```python
from build123d import *

# Parameters (mm, degrees)
BOSS_EXTRUDE1_DEPTH = 5
CUT_EXTRUDE1_DEPTH  = 2


with BuildPart() as part:
    # Sketch1 → Boss-Extrude1 (new body)
    with BuildSketch(Plane.XY):
        Polygon((-73.645107518, -74.864510752), (-51.383851785, -74.864510752), (-51.383851785, -79.864510752), (-31.383851785, -79.864510752), (-31.383851785, -74.864510752), (22.715789763, -74.864510752), (22.715789763, -79.864510752), (42.715789763, -79.864510752), (42.715789763, -74.864510752), (76.354892482, -74.864510752), (76.354892482, -60.328664174), (71.354892482, -60.328664174), (71.354892482, -40.328664174), (76.354892482, -40.328664174), (76.354892482, -12.973595237), (71.354892482, -12.973595237), (71.354892482, 7.026404763), (76.354892482, 7.026404763), (76.354892482, 37.571193369), (71.355899646, 37.470840861), (71.355899646, 57.470840861), (76.354892482, 57.571193369), (76.354892482, 75.135489248), (42.715789763, 75.135489248), (42.715789763, 80.135489248), (22.715789763, 80.135489248), (22.715789763, 75.135489248), (-31.383851785, 75.135489248), (-31.383851785, 80.135489248), (-51.383851785, 80.135489248), (-51.383851785, 75.135489248), (-73.645107518, 75.135489248), (-73.645107518, 57.571193369), (-68.646114682, 57.470840861), (-68.646114682, 37.470840861), (-73.645107518, 37.571193369), (-73.645107518, 7.026404763), (-68.645107518, 7.026404763), (-68.645107518, -12.973595237), (-73.645107518, -12.973595237), (-73.645107518, -40.328664174), (-68.645107518, -40.328664174), (-68.645107518, -60.328664174), (-73.645107518, -60.328664174), align=None)
    extrude(amount=BOSS_EXTRUDE1_DEPTH)

    # Sketch2 → Cut-Extrude1 (cut)
    with BuildSketch(Plane.XY.offset(5)):
        with BuildLine():
            Line((-24.19666878, 43.178385546), (-25.33641237, 43.178385546))
            add(Edge.make_bspline(
                [(-25.33641237, 43.178385546), (-25.328984129, 43.329591339), (-25.314395262, 43.626555492), (-25.246075469, 44.059530809), (-25.148318572, 44.473386793), (-25.01010101, 44.864800481), (-24.838446802, 45.237232725), (-24.632597846, 45.58920421), (-24.38878016, 45.919372238), (-24.112258582, 46.22467604), (-23.811926663, 46.504756655), (-23.487873683, 46.746619964), (-23.147350298, 46.950972657), (-22.791389622, 47.121810306), (-22.415975577, 47.250043461), (-22.024514921, 47.345190554), (-21.615287769, 47.402436151), (-21.33646826, 47.40858943), (-21.194665575, 47.41171888)],
                knots=[0, 0, 0, 0, 0.000453872, 0.000891393, 0.001312835, 0.001728009, 0.002134376, 0.002541468, 0.002949043, 0.00336336, 0.003775633, 0.004179123, 0.004573978, 0.004965443, 0.005361289, 0.005761752, 0.006172633, 0.006597866, 0.006597866, 0.006597866, 0.006597866], degree=3))
            add(Edge.make_bspline(
                [(-21.194665575, 47.41171888), (-21.055407992, 47.408458766), (-20.781771816, 47.40205276), (-20.382403935, 47.347039882), (-20.002212038, 47.260877307), (-19.641939285, 47.139989939), (-19.304460136, 46.977486445), (-18.987239375, 46.782278234), (-18.686500433, 46.556509131), (-18.415784389, 46.290702437), (-18.16719793, 46.006939499), (-17.952741176, 45.703997677), (-17.769087697, 45.391108555), (-17.616006687, 45.065886223), (-17.503317269, 44.725268492), (-17.417762057, 44.374214356), (-17.369402584, 44.009090042), (-17.361980619, 43.76196054), (-17.358207242, 43.636318239)],
                knots=[0, 0, 0, 0, 0.000417607, 0.000820584, 0.001206914, 0.001585844, 0.001957948, 0.002327951, 0.002701938, 0.003083379, 0.003463911, 0.003832406, 0.004194997, 0.004551257, 0.004908462, 0.005269442, 0.005633919, 0.006010863, 0.006010863, 0.006010863, 0.006010863], degree=3))
            add(Edge.make_bspline(
                [(-17.358207242, 43.636318239), (-17.364327354, 43.459426074), (-17.376460178, 43.108745951), (-17.481165156, 42.592747282), (-17.642934479, 42.092348925), (-17.839142328, 41.689653506), (-18.037336959, 41.366794494), (-18.212160789, 41.09858631), (-18.421356469, 40.812559028), (-18.66300994, 40.505831861), (-18.933475694, 40.177466576), (-19.234700346, 39.827328424), (-19.568984994, 39.459136174), (-19.803601825, 39.207655081), (-19.925174389, 39.07734388)],
                knots=[0, 0, 0, 0, 0.000530199, 0.001051094, 0.001573224, 0.002104594, 0.002389938, 0.002709581, 0.003064778, 0.003452579, 0.003880929, 0.004340927, 0.00483807, 0.005372718, 0.005372718, 0.005372718, 0.005372718], degree=3))
            Line((-19.925174389, 39.07734388), (-23.10271846, 35.688641956))
            Line((-23.10271846, 35.688641956), (-17.195386729, 35.688641956))
            Line((-17.195386729, 35.688641956), (-17.195386729, 34.386077854))
            Line((-17.195386729, 34.386077854), (-25.824873909, 34.386077854))
            Line((-25.824873909, 34.386077854), (-20.899553396, 39.642127533))
            add(Edge.make_bspline(
                [(-20.899553396, 39.642127533), (-20.779636778, 39.767307103), (-20.549301497, 40.007751437), (-20.223519004, 40.358790178), (-19.930914675, 40.684452798), (-19.669594421, 40.984123988), (-19.44522713, 41.262187105), (-19.246119317, 41.509636458), (-19.08658703, 41.737345463), (-18.913448308, 42.001289977), (-18.745757576, 42.323551813), (-18.601658455, 42.717374057), (-18.513793148, 43.122784374), (-18.503252745, 43.396748909), (-18.497950832, 43.534555418)],
                knots=[0, 0, 0, 0, 0.000520043, 0.000998896, 0.001436661, 0.001833471, 0.002191472, 0.002508543, 0.002785952, 0.003025175, 0.003455296, 0.003872183, 0.004280329, 0.004693418, 0.004693418, 0.004693418, 0.004693418], degree=3))
            add(Edge.make_bspline(
                [(-18.497950832, 43.534555418), (-18.500257668, 43.621210778), (-18.504803999, 43.791991852), (-18.544927645, 44.042384178), (-18.60556291, 44.283919359), (-18.692449989, 44.517340349), (-18.807137303, 44.740300286), (-18.94674071, 44.953070571), (-19.107813226, 45.158770531), (-19.294144974, 45.35164107), (-19.498838203, 45.528284301), (-19.715080195, 45.684763125), (-19.943862002, 45.815533613), (-20.184219016, 45.922734303), (-20.435481148, 46.006827829), (-20.698134366, 46.065097531), (-20.97145294, 46.101682544), (-21.158083053, 46.10663254), (-21.253179197, 46.109154777)],
                knots=[0, 0, 0, 0, 0.000259807, 0.000512029, 0.000758843, 0.001005985, 0.001257437, 0.001509351, 0.001768409, 0.002040101, 0.00231246, 0.002578628, 0.002839591, 0.003101519, 0.003367006, 0.003633016, 0.003907552, 0.004192772, 0.004192772, 0.004192772, 0.004192772], degree=3))
            add(Edge.make_bspline(
                [(-21.253179197, 46.109154777), (-21.352496219, 46.106560231), (-21.547538451, 46.101464972), (-21.833901799, 46.065822734), (-22.10708162, 46.004333542), (-22.367765097, 45.920235323), (-22.616393308, 45.813342875), (-22.851757125, 45.680204258), (-23.07332818, 45.521332726), (-23.281522993, 45.341208422), (-23.473343717, 45.140665983), (-23.641879524, 44.917109831), (-23.789141518, 44.674621781), (-23.917626451, 44.413856126), (-24.021968527, 44.132446696), (-24.101699673, 43.831392453), (-24.164789088, 43.512000583), (-24.18586572, 43.291437561), (-24.19666878, 43.178385546)],
                knots=[0, 0, 0, 0, 0.000297928, 0.000585081, 0.00086406, 0.001136798, 0.001405713, 0.001674567, 0.001946354, 0.002222301, 0.00249943, 0.002777246, 0.003060416, 0.003349412, 0.003648067, 0.00395911, 0.004282927, 0.004623434, 0.004623434, 0.004623434, 0.004623434], degree=3))
        make_face()
    extrude(amount=-CUT_EXTRUDE1_DEPTH, mode=Mode.SUBTRACT)


solid = part.part
```
Check sheet for the modelled part. Datum: model origin and axes. Units: mm. A direction names the side the tool comes from. Round coordinates to 2 decimals unless told otherwise and drop trailing zeros. Write each loop counter-clockwise with the first axis right and the second up, starting at its lowest first coordinate (ties: lowest second). Pieces come first, ordered by that corner, then holes. Notation, with made-up numbers: (75, -0.5) -> (116, -0.5) arc R28 ccw to (116, 25.5) -> close; hole circle Ø9 at (71, 33.5). An arc over 180 degrees is marked (long way). One line per question, with ' | ' between items. Start each with the question number.
1. Release check for a two-part mould opening along Y. For faces 1 (the face through (-73.645, -67, 2)), 2 (the face through (74, 7.026, 2)), 3 (the face through (-42, -79.865, 2)) record: +Y half, -Y half, draft (parallel to the pull), parting line (faces both ways), or undercut.
2. Sectioned sample at A-A, the plane x = 6. Record the cut outline in (y, z), then the cut area to 3 significant figures.
3. Set-up check for faces 4 (the face through (59, -74.865, 2)), 5 (the face through (71.355, -50, 2)), 6 (the face through (-31.384, 78, 2)): record each of +Z, -Z, +X, -X, +Y, -Y from which the full face is reachable in a straight line by a thin tool's end or side.
4. Sectioned sample at B-B, the plane y = 53. Record the cut outline in (x, z).
5. Depth check by flat-ended pin: pin 1 (2 mm diameter, centred on x = -20, z = 3.5, fed in from -Y); pin 2 (2.5 mm diameter, centred on y = 76.5, z = 2, fed in from -X); pin 3 (1.5 mm diameter, centred on x = 67.5, z = 1.5, fed in from +Y). Enter the tip coordinate at first touch or a pass-through.
6. Scan lines: line 1 along Y through (x, z) = (-16.5, 0.3); line 2 along X through (y, z) = (-5.5, 2.45). Record each from-to range of solid material in increasing order. Write a range as from..to.
Taken from the geometry:
1) face 1: draft | face 2: undercut | face 3: -Y half
2) outline: (-74.86, 0) -> (75.14, 0) -> (75.14, 5) -> (-74.86, 5) -> close | area: 750 mm^2
3) face 4: +Z, -Z, +X, -Y | face 5: +Z, -Z, +X | face 6: +Z, -Z, +Y
4) outline: (-68.65, 0) -> (71.36, 0) -> (71.36, 5) -> (-68.65, 5) -> close
5) pin 1: stops at y = -74.86 | pin 2: stops at x = -51.38 | pin 3: stops at y = 75.14
6) line 1: y = -74.86..75.14 | line 2: x = -68.65..71.35
